from build123d import *

# Parameters (mm, degrees)
SKETCH1_R           = 4
BOSS_EXTRUDE1_DEPTH = 157.5
CHAMFER1_SIZE       = 0.5
SKETCH2_R           = 1.65
CUT_EXTRUDE1_DEPTH  = 12
CUT_EXTRUDE2_START  = -12
SKETCH3_R           = 1.65
CUT_EXTRUDE2_DEPTH  = 12


with BuildPart() as part:
    # Sketch1 → Boss-Extrude1 (new, symmetric)
    with BuildSketch(Plane(origin=(0, 0, 0), x_dir=(1, 0, 0), z_dir=(0, 1, 0))):
        with Locations(Location((0, 0, 0), (0, 0, 270))):
            Circle(SKETCH1_R)
    extrude(amount=BOSS_EXTRUDE1_DEPTH, both=True)

    # Chamfer1
    chamfer1_edges = [part.edges().sort_by_distance(p)[0] for p in [
        (0, -157.5, -4),
        (0, 157.5, -4),
    ]]
    chamfer(chamfer1_edges, length=CHAMFER1_SIZE)

    # Sketch2 → Cut-Extrude1 (cut)
    with BuildSketch(Plane(origin=(0, 157.5, 0), x_dir=(1, 0, 0), z_dir=(0, 1, 0))):
        with Locations(Location((0, 0, 0), (0, 0, 270))):
            Circle(SKETCH2_R)
    extrude(amount=-CUT_EXTRUDE1_DEPTH, mode=Mode.SUBTRACT)

    # Sketch3 → Cut-Extrude2 (cut)
    with BuildSketch(Plane.XZ.offset(157.5).offset(CUT_EXTRUDE2_START)):
        with Locations(Location((0, 0, 0), (0, 0, 90))):
            Circle(SKETCH3_R)
    extrude(amount=CUT_EXTRUDE2_DEPTH, mode=Mode.SUBTRACT)


solid = part.part
CAD build for the part. Positions are in the model's coordinates, mm. Coordinates: 2 decimals unless noted, no trailing zeros. Write each loop counter-clockwise with the first axis right and the second up, starting at its lowest first coordinate (ties: lowest second). Pieces come first, ordered by that corner, then holes. Notation, with made-up numbers: (-38.5, -17.5) - (10.5, -17.5) arc R20 ccw to (10.5, 17.5) - close; hole circle Ø11 at (16.25, 89.5). An arc over 180 degrees is marked (long way). Use a Markdown table: item, result. Add a question column.
Item 1: Flat gauge pins, fed straight in: pin 1 (1.6 mm diameter, centred on x = 0.5, z = 0, fed in from -Y); pin 2 (4 mm diameter, centred on x = 2.5, y = 106.5, fed in from +Z); pin 3 (1.5 mm diameter, centred on x = 3, y = -31, fed in from -Z). Where does each tip first touch, or does it go through?
Item 2: Band-saw the part on B-B, the plane z = 0. Give the cut face in (x, y), and give its area (3 significant figures).
Item 3: Band-saw the part on A-A, the plane x = 0. Give the cut face in (y, z), and give its area (3 significant figures).
Item 4: Band-saw the part on C-C, the plane y = -115. Give the cut face in (x, z), and give its area (3 significant figures).
Item 5: Drill centre lines: L1, parallel to X at y = 148.5, z = 0; L2, parallel to Z at x = -0.5, y = 101; L3, parallel to X at y = 94, z = -0.25. Where is each one in solid material? Low to high. Write a range as from..to.
Numbers:
| question | item | result |
|---|---|---|
| 1 | pin 1 | y = -145.5 |
| 1 | pin 2 | z = 3.97 |
| 1 | pin 3 | z = -3.31 |
| 2 | outline | (-4, -157) - (-3.5, -157.5) - (-1.65, -157.5) - (-1.65, -145.5) - (1.65, -145.5) - (1.65, -157.5) - (3.5, -157.5) - (4, -157) - (4, 157) - (3.5, 157.5) - (1.65, 157.5) - (1.65, 145.5) - (-1.65, 145.5) - (-1.65, 157.5) - (-3.5, 157.5) - (-4, 157) - close |
| 2 | area | 2,440 mm2 |
| 3 | outline | (-157.5, -3.5) - (-157, -4) - (157, -4) - (157.5, -3.5) - (157.5, -1.65) - (145.5, -1.65) - (145.5, 1.65) - (157.5, 1.65) - (157.5, 3.5) - (157, 4) - (-157, 4) - (-157.5, 3.5) - (-157.5, 1.65) - (-145.5, 1.65) - (-145.5, -1.65) - (-157.5, -1.65) - close |
| 3 | area | 2,440 mm2 |
| 4 | outline | circle Ø8 at (0, 0) |
| 4 | area | 50.3 mm2 |
| 5 | L1 | -4..-1.65, 1.65..4 |
| 5 | L2 | -3.97..3.97 |
| 5 | L3 | -3.99..3.99 |
